Design review of the part built by this model. Coordinates are the model's own, in mm. A direction names the side the tool comes from. Give positions to 0.01 mm unless a question says otherwise; leave off trailing zeros. Write each loop counter-clockwise with the first axis right and the second up, starting at its lowest first coordinate (ties: lowest second). Pieces come first, ordered by that corner, then holes. Notation, with made-up numbers: M -6.5,40 L 42.5,40 A8 ccw 42.5,53 Z; hole C 84.5,55 d9. An arc over 180 degrees is marked long. Answer in a Markdown table with one row per item.
```python
from build123d import *

# Parameters (mm, degrees)
BOSS_EXTRUDE2_DEPTH = 7
BOSS_EXTRUDE3_DEPTH = 15


with BuildPart() as part:
    # Sketch1 → Boss-Extrude2 (new body)
    with BuildSketch(Plane.XY):
        with BuildLine():
            Line((-40.843938812, -25.02529653), (21.822672825, -14.817519442))
            Line((21.822672825, -14.817519442), (26.489801196, 7.266810726))
            Line((26.489801196, 7.266810726), (34.744303123, 7.266810726))
            Line((34.744303123, 7.266810726), (34.744303123, 11.354641566))
            Line((34.744303123, 11.354641566), (23.2245968, 11.838054321))
            Line((23.2245968, 11.838054321), (22.594616957, 29.052034329))
            Line((22.594616957, 29.052034329), (9.094616957, 29.052034329))
            Line((9.094616957, 29.052034329), (9.094616957, 2.846901584))
            ThreePointArc((9.094616957, 2.846901584), (4.094616957, -2.153098416), (-0.905383043, 2.846901584))
            Line((-0.905383043, 2.846901584), (-0.905383043, 20.539136331))
            Line((-0.905383043, 20.539136331), (-10.036820206, 32.783811613))
            Line((-10.036820206, 32.783811613), (-20.38656022, 37.570023616))
            Line((-20.38656022, 37.570023616), (-22.572356812, 32.843440998))
            Line((-22.572356812, 32.843440998), (-36.411901157, 38.132027383))
            Line((-36.411901157, 38.132027383), (-40.843938812, 1.825568171))
            Line((-40.843938812, 1.825568171), (-40.843938812, -25.02529653))
        make_face()
    extrude(amount=BOSS_EXTRUDE2_DEPTH)

    # Sketch1<7> → Boss-Extrude3 (add)
    with BuildSketch(Plane.XY):
        with BuildLine():
            ThreePointArc((-3.054484565, 16.834095496), (-1.998003486, 17.361409284), (-0.905383043, 17.809061684))
            Line((-0.905383043, 17.809061684), (-0.905383043, 20.539136331))
            Line((-0.905383043, 20.539136331), (-10.036820206, 32.783811613))
            Line((-10.036820206, 32.783811613), (-20.38656022, 37.570023616))
            Line((-20.38656022, 37.570023616), (-22.572356812, 32.843440998))
            Line((-22.572356812, 32.843440998), (-12.451357463, 28.975844058))
            Line((-12.451357463, 28.975844058), (-3.054484565, 16.834095496))
        make_face()
        with BuildLine():
            ThreePointArc((20.523303512, 3.077207951), (16.644968484, -7.575511067), (6.665935601, -12.955177206))
            Line((6.665935601, -12.955177206), (-40.843938812, -20.694070291))
            Line((-40.843938812, -20.694070291), (-40.843938812, -25.02529653))
            Line((-40.843938812, -25.02529653), (21.822672825, -14.817519442))
            Line((21.822672825, -14.817519442), (26.489801196, 7.266810726))
            Line((26.489801196, 7.266810726), (34.744303123, 7.266810726))
            Line((34.744303123, 7.266810726), (34.744303123, 11.354641566))
            Line((34.744303123, 11.354641566), (23.2245968, 11.838054321))
            Line((23.2245968, 11.838054321), (22.257186267, 10.122973627))
            Line((22.257186267, 10.122973627), (20.850125794, 5.080010211))
            Line((20.850125794, 5.080010211), (20.523303512, 3.077207951))
        make_face()
        with BuildLine():
            Line((-26.832821067, 18.003435216), (-40.843938812, 23.904400779))
            Line((-40.843938812, 23.904400779), (-40.843938812, 0.147997265))
            Line((-40.843938812, 0.147997265), (-26.961449929, 4.612329337))
            ThreePointArc((-26.961449929, 4.612329337), (-22.405428772, 11.264736988), (-26.832821067, 18.003435216))
        make_face()
    extrude(amount=BOSS_EXTRUDE3_DEPTH)


solid = part.part
```
1) The part is to be moulded in two halves that separate along Y. For faces 6 (the face through (-10, -20, 7)), 7 (the face through (2, -15, 15)), 8 (the face through (22.914, 20.325, 3.451)), 9 (the face through (-34, 2.35, 10.94)), say which applies: released by +Y, released by -Y, zero draft, split by the parting line, or undercut.
Geometry says:
| item | result |
|---|---|
| face 6 | released by -Y |
| face 7 | zero draft |
| face 8 | released by +Y |
| face 9 | undercut |
2) To check wall thickness, follow probe 1 along X at (y, z) = (23, 1.75); probe 2 along Z at (x, y) = (-19, 19.5); probe 3 along X at (y, z) = (14, 2). State the ranges of each line that lie inside material, in increasing order. Write a range as [from, to].
Geometry says:
| item | result |
|---|---|
| probe 1 | [-40.84, -38.7], [-38.26, -2.74], [9.09, 22.82] |
| probe 2 | [0, 7] |
| probe 3 | [-40.84, -0.91], [9.09, 23.15] |
3) Insertion check: P1, Ø1.5, axis at x = 7.5, z = 13, coming from the +Y side; P2, Ø2, axis at x = 16, z = 5, coming from the +Y side. Each pin has a flat end and moves straight along its axis. Give the tip position at first contact, or say it passes through.
Geometry says:
| item | result |
|---|---|
| P1 | y = -12.66 |
| P2 | y = 29.05 |
4) Add section D-D (y = 34). Write out the cut boundary in (x, z), and give its area (3 significant figures).
Geometry says:
| item | result |
|---|---|
| outline | M -36.92,0 L -25.6,0 L -25.6,7 L -36.92,7 Z; M -22.04,0 L -12.67,0 L -12.67,15 L -22.04,15 Z |
| area | 220 mm^2 |
5) Add section C-C (x = -19). Write out the cut boundary in (y, z), and give its area (3 significant figures).
Geometry says:
| item | result |
|---|---|
| outline | M -21.47,0 L 36.93,0 L 36.93,15 L 31.48,15 L 31.48,7 L -17.14,7 L -17.14,15 L -21.47,15 Z |
| area | 487 mm^2 |
6) For faces 1 (the face through (16, 29.052, 3)), 2 (the face through (-16.76, -16.77, 10.94)), 3 (the face through (-35.3, 21.57, 9.06)), 4 (the face through (-21.464, 35.24, 7.395)), 5 (the face through (31, 7.267, 7)), list the 3-axis set-ups (+Z, -Z, +X, -X, +Y, -Y) from which the entire face can be reached by the end or side of a thin tool; tool diameter is ignored.
Geometry says:
| item | result |
|---|---|
| face 1 | +Z, -Z, +X, +Y |
| face 2 | +Z, -X |
| face 3 | +Z, +Y |
| face 4 | +Z, -Z, +Y |
| face 5 | +Z, -Z, +X, -Y |
7) Add section A-A (z = 13). Write out the cut boundary in (x, y), and give its area (3 significant figures).
Geometry says:
| item | result |
|---|---|
| outline | M -40.84,-25.03 L 21.82,-14.82 L 26.49,7.27 L 34.74,7.27 L 34.74,11.35 L 23.22,11.84 L 22.26,10.12 L 20.85,5.08 L 20.52,3.08 A15.94 cw 6.67,-12.96 L -40.84,-20.69 Z; M -40.84,0.15 L -26.96,4.61 A7.24 ccw -26.83,18 L -40.84,23.9 Z; M -22.57,32.84 L -12.45,28.98 L -3.05,16.83 A15.94 cw -0.91,17.81 L -0.91,20.54 L -10.04,32.78 L -20.39,37.57 Z |
| area | 858 mm^2 |
8) Add section B-B (y = 15.5). Write out the cut boundary in (x, z).
Geometry says:
| item | result |
|---|---|
| outline | M -40.84,0 L -0.91,0 L -0.91,7 L -23.72,7 L -23.72,15 L -40.84,15 Z; M 9.09,0 L 23.09,0 L 23.09,7 L 9.09,7 Z |
